CAD build for the part. Positions are in the model's coordinates, mm. A direction names the side the tool comes from. Give positions to 0.01 mm unless a question says otherwise; leave off trailing zeros. Write each loop counter-clockwise with the first axis right and the second up, starting at its lowest first coordinate (ties: lowest second). Pieces come first, ordered by that corner, then holes. Notation, with made-up numbers: (3, 26.25) - (23, 26.25) arc R13 ccw to (23, 43.25) - close; hole circle Ø3 at (-33.75, -17.75). An arc over 180 degrees is marked (long way). Answer as a JSON object with one key per item and string values.
Autodesk Inventor part; units mm, degrees
ref_plane "YZ Plane" through (0, 0, 0) normal (1, 0, 0) x (0, 1, 0)
ref_plane "XZ Plane" through (0, 0, 0) normal (0, 1, 0) x (-1, 0, 0)
ref_plane "XY Plane" through (0, 0, 0) normal (0, 0, 1) x (1, 0, 0)
sketch "Эскиз1" plane through (0, 0, 0) normal (0, 0, 1) x (1, 0, 0)
  line L0 (-3, 7.5) -> (3, 7.5)
  line L1 (3, 7.5) -> (3, -7.5)
  line L2 (3, -7.5) -> (-3, -7.5)
  line L3 (-3, -7.5) -> (-3, 7.5)
  point P0 (0, 0)
  point P1 (3, 0)
  point P2 (0, 7.5)
  dimension "d0" = 6
  dimension "d1" = 15
extrude "Выдавливание1" add sketch "Эскиз1" along normal blind 3
sketch "Эскиз2" plane through (0, 0, 3) normal (0, 0, 1) x (1, 0, 0)
  line L0 (3, 7.5) -> (-3, 7.5)
  point P0 (0, 0)
  point P1 (0, 0)
  dimension "d4" = 7.5
hole "Отверстие1" at (0, 0, 3) direction (0, 0, -1) diameter 3 end through all
sketch "Эскиз3" plane through (0, 0, 3) normal (0, 0, 1) x (1, 0, 0)
  line L0 (3, -7.5) -> (3, 7.5)
  line L1 (-3, -7.5) -> (3, -7.5)
  line L2 (3, -7.5) -> (3, -4.5)
  line L3 (3, -4.5) -> (-3, -4.5)
  line L4 (-3, -4.5) -> (-3, -7.5)
  dimension "d12" = 3
extrude "Выдавливание2" add sketch "Эскиз3" along normal blind 9
properties part number "Угловой_крепеж"
Item 1: Cut at A-A (x = 0). Give the cut face in (y, z).
Entries:
{"outline": "(-7.5, 0) - (-1.5, 0) - (-1.5, 3) - (-4.5, 3) - (-4.5, 12) - (-7.5, 12) - close; (1.5, 0) - (7.5, 0) - (7.5, 3) - (1.5, 3) - close"}
Item 2: Mould opens along Y. For faces 1 (the cylindrical face through (-0.07, 1.5, 1.48)), 2 (the flat face through (0, 7.5, 1)), 3 (the flat face through (0, -7.5, 6)), 4 (the flat face through (0, -6, 12)) say: +Y half, -Y half, draft (parallel to the pull), parting line (faces both ways), or undercut.
Entries:
{"face 1": "undercut", "face 2": "+Y half", "face 3": "-Y half", "face 4": "draft"}
Item 3: Cut at B-B (y = 0). Give the cut face in (x, z), and give its area (3 significant figures).
Entries:
{"outline": "(-3, 0) - (-1.5, 0) - (-1.5, 3) - (-3, 3) - close; (1.5, 0) - (3, 0) - (3, 3) - (1.5, 3) - close", "area": "9.00 mm2"}
Item 4: Cut at C-C (x = 2.5). Give the cut face in (y, z), and give its area (3 significant figures).
Entries:
{"outline": "(-7.5, 0) - (7.5, 0) - (7.5, 3) - (-4.5, 3) - (-4.5, 12) - (-7.5, 12) - close", "area": "72.0 mm2"}
Item 5: Flat gauge pins, fed straight in: P1, Ø3, axis at x = 2.5, z = 8, coming from the +Y side; P2, Ø1.8, axis at x = 0, y = 0, coming from the -Z side; P3, Ø1.5, axis at x = 2.5, y = -1.5, coming from the +Z side. Where does each tip first touch, or does it go through?
Entries:
{"P1": "y = -4.5", "P2": "through", "P3": "z = 3"}
Item 6: Cut at D-D (y = 2.5). Give the cut face in (x, z).
Entries:
{"outline": "(-3, 0) - (3, 0) - (3, 3) - (-3, 3) - close"}
Item 7: Probe line 1 (X direction, y = 0, z = 0.8); line 2 (Y direction, x = 0, z = 1.6); line 3 (Y direction, x = 2.45, z = 5.25). List the from-to ranges inside material, lowest first. Write a range as from..to.
Entries:
{"line 1": "-3..-1.5, 1.5..3", "line 2": "-7.5..-1.5, 1.5..7.5", "line 3": "-7.5..-4.5"}
Item 8: Which spindle directions (+Z, -Z, +X, -X, +Y, -Y) get a long thin tool onto all of the face, cutting with end or side? Do faces 5 (the flat face through (-3, -3, 2)), 6 (the flat face through (0, -4.5, 7)). Say none if no direction does.
Entries:
{"face 5": "+Z, -Z, -X, +Y, -Y", "face 6": "+Z, +X, -X, +Y"}
